Check sheet for the drawn part. Datum: minimum x, y, z corner. Units: mm. A direction names the side the tool comes from. Coordinates: 2 decimals unless noted, no trailing zeros. Order: outer loops, then holes, each group sorted by start corner. A loop starts at its lowest first (then second) coordinate and runs counter-clockwise, first axis right, second up. Notation, with made-up numbers: (29, 32) - (43, 32) arc R21 cw to (43, 36) - close; hole circle Ø7 at (38, -23.75). An arc over 180 degrees is marked (long way). Put each result on its own line as item: value.
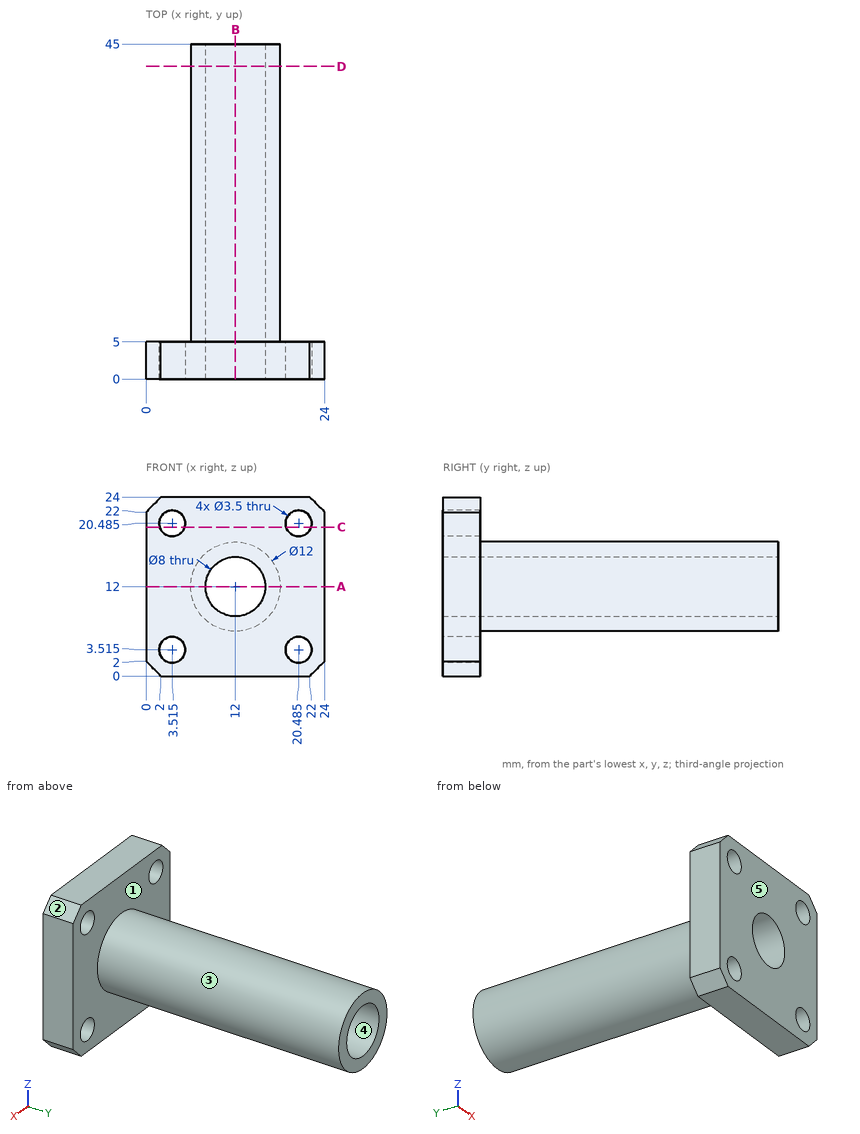
Q1. Depth check by flat-ended pin: pin 1 Ø10 at (x, y) = (12, 23.5) entering from +Z; pin 2 Ø4 at (x, z) = (3.51, 20.49) entering from +Y; pin 3 Ø12 at (x, y) = (9, 34) entering from -Z; pin 4 Ø10.5 at (x, z) = (12, 12) entering from +Y. Enter the tip coordinate at first touch or a pass-through.
Answer block:
pin 1: stops at z = 18
pin 2: stops at y = 5
pin 3: stops at z = 6
pin 4: stops at y = 45
Q2. Section check B-B on x = 12. Record the boundary of the cut face in (y, z), then the cut area to 3 significant figures.
Answer block:
outline: (0, 0) - (5, 0) - (5, 6) - (45, 6) - (45, 8) - (0, 8) - close; (0, 16) - (45, 16) - (45, 18) - (5, 18) - (5, 24) - (0, 24) - close
area: 240 mm^2
Q3. Draft check along X on the marked faces 3, 4 and 5. Enter one of: pulls with the +X half, pulls with the -X half, needs draft (parallel to the pull), parting line crosses it, or undercut.
Answer block:
face 3: parting line crosses it
face 4: undercut
face 5: needs draft
Q4. Section check A-A on z = 12. Record the boundary of the cut face in (x, y), then the cut area to 3 significant figures.
Answer block:
outline: (0, 0) - (8, 0) - (8, 45) - (6, 45) - (6, 5) - (0, 5) - close; (16, 0) - (24, 0) - (24, 5) - (18, 5) - (18, 45) - (16, 45) - close
area: 240 mm^2
Q5. Thickness scan on L1, parallel to Z at x = 12, y = 31; L2, parallel to Y at x = 16.75, z = 20.5; L3, parallel to Z at x = 13, y = 12. Record the ranges inside material, lowest first. Write a range as [from, to].
Answer block:
L1: z = [6, 8], [16, 18]
L2: y = [0, 5]
L3: z = [6.08, 8.13], [15.87, 17.92]
Q6. Section check D-D on y = 42. Record the boundary of the cut face in (x, z).
Answer block:
outline: circle Ø12 at (12, 12); hole circle Ø8 at (12, 12)
Q7. Section check C-C on z = 20. Record the boundary of the cut face in (x, y).
Answer block:
outline: (0, 0) - (1.83, 0) - (1.83, 5) - (0, 5) - close; (5.2, 0) - (18.8, 0) - (18.8, 5) - (5.2, 5) - close; (22.17, 0) - (24, 0) - (24, 5) - (22.17, 5) - close
Q8. Access from +Z, -Z, +X, -X, +Y, -Y to the whole of each face (thin tool, end or side, straight path). Record for the marked faces 1 and 2.
Answer block:
face 1: +Y
face 2: +Z, +X, +Y, -Y
